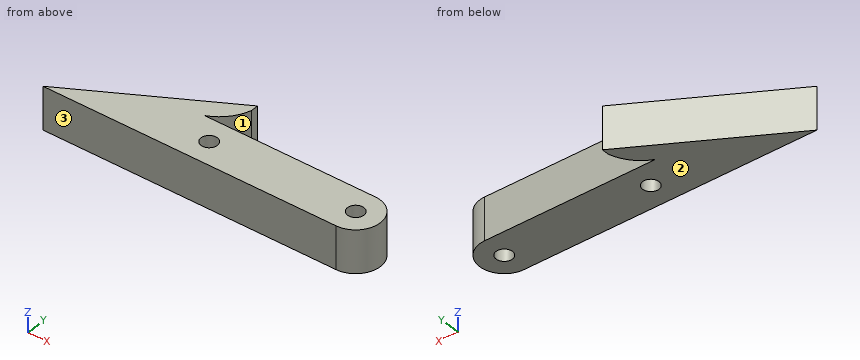
from build123d import *

# Parameters (mm, degrees)
SKETCH1_R           = 2.5
BOSS_EXTRUDE1_DEPTH = 6.5


with BuildPart() as part:
    # Sketch1 → Boss-Extrude1 (new, symmetric)
    with BuildSketch(Plane.XY):
        with BuildLine():
            ThreePointArc((22.5, -7.5), (30, 0), (22.5, 7.5))
            Line((22.5, 7.5), (-30, 7.5))
            ThreePointArc((-30, 7.5), (-25.225001549, 10.954803468), (-22.5, 16.180762114))
            Line((-22.5, 16.180762114), (-22.5, 18.480762114))
            Line((-22.5, 18.480762114), (-67.5, -7.5))
            Line((-67.5, -7.5), (22.5, -7.5))
        make_face()
        with Locations((-22.5, 0)):
            Circle(SKETCH1_R, mode=Mode.SUBTRACT)
        with Locations((22.5, 0)):
            Circle(SKETCH1_R, mode=Mode.SUBTRACT)
    extrude(amount=BOSS_EXTRUDE1_DEPTH, both=True)


solid = part.part
Could you check a few things on this model? Use its own coordinates, in mm. Face numbers are marked on the shaded views. Give positions to 0.01 mm unless a question says otherwise; leave off trailing zeros. Order: outer loops, then holes, each group sorted by start corner. A loop starts at its lowest first (then second) coordinate and runs counter-clockwise, first axis right, second up. Notation, with made-up numbers: (-28.75, 55) -> (-18.75, 55) arc R22 cw to (-18.75, 86) -> close; hole circle Ø10 at (73.25, 15.25). An arc over 180 degrees is marked (long way). Answer in a Markdown table with one row per item. Add a question column.
Item 1: Imagine slicing it at C-C (x = 15.5). List the corners of the cut face in (y, z) for me.
Item 2: Imagine slicing it at B-B (y = 0). List the corners of the cut face in (x, z) for me, and give its area (3 significant figures).
Item 3: Imagine slicing it at D-D (y = 8.75). List the corners of the cut face in (x, z) for me, and give its area (3 significant figures).
Item 4: I'm going to push flat-ended pins straight in: P1, Ø4, axis at x = -22.5, y = 0, coming from the +Z side; P2, Ø6, axis at y = -0.5, z = 0, coming from the -X side; P3, Ø1.8, axis at y = 17, z = 1.5, coming from the +X side. Where does each tip first touch, or does it pass through?
Item 5: We'd pull the mould along Y, two halves only. Please class the marked faces 1, 2 and 3: pulls with the +Y half, pulls with the -Y half, needs draft (parallel to the pull), parting line crosses it, or undercut.
Item 6: Imagine slicing it at A-A (z = -2.5). List the corners of the cut face in (x, y) for me, and give its area (3 significant figures).
Item 7: Please list where these lines run through material, in increasing order: probe 1 along Y at (x, z) = (22.5, -3.5); probe 2 along X at (y, z) = (0.5, 6); probe 3 along Y at (x, z) = (-21, 2).
Result:
| question | item | result |
|---|---|---|
| 1 | outline | (-7.5, -6.5) -> (7.5, -6.5) -> (7.5, 6.5) -> (-7.5, 6.5) -> close |
| 2 | outline | (-54.51, -6.5) -> (-25, -6.5) -> (-25, 6.5) -> (-54.51, 6.5) -> close; (-20, -6.5) -> (20, -6.5) -> (20, 6.5) -> (-20, 6.5) -> close; (25, -6.5) -> (30, -6.5) -> (30, 6.5) -> (25, 6.5) -> close |
| 2 | area | 969 mm2 |
| 3 | outline | (-39.35, -6.5) -> (-27.69, -6.5) -> (-27.69, 6.5) -> (-39.35, 6.5) -> close |
| 3 | area | 152 mm2 |
| 4 | P1 | through |
| 4 | P2 | x = -60.57 |
| 4 | P3 | x = -22.5 |
| 5 | face 1 | undercut |
| 5 | face 2 | needs draft |
| 5 | face 3 | pulls with the -Y half |
| 6 | outline | (-67.5, -7.5) -> (22.5, -7.5) arc R7.5 ccw to (22.5, 7.5) -> (-30, 7.5) arc R12.82 ccw to (-22.5, 16.18) -> (-22.5, 18.48) -> close; hole circle Ø5 at (-22.5, 0); hole circle Ø5 at (22.5, 0) |
| 6 | area | 1,290 mm2 |
| 7 | probe 1 | -7.5 to -2.5, 2.5 to 7.5 |
| 7 | probe 2 | -53.64 to -24.95, -20.05 to 20.05, 24.95 to 29.98 |
| 7 | probe 3 | -7.5 to -2, 2 to 7.5 |
